from build123d import *

# Parameters (mm, degrees)
BOSS_EXTRUDE4_DEPTH                                 = 50
CBORE_FOR_00_BINDING_HEAD_MACHINE_SCREW_D           = 10.000000066
CBORE_FOR_00_BINDING_HEAD_MACHINE_SCREW_CBORE_D     = 19.999999878
CBORE_FOR_00_BINDING_HEAD_MACHINE_SCREW_CBORE_DEPTH = 3.000000096
BOSS_EXTRUDE5_REACH                                 = 119.883
SKETCH13_W                                          = 50
SKETCH13_H                                          = 2.915477917
BOSS_EXTRUDE5_DIRECTION_2_REACH                     = 119.883
CUT_EXTRUDE4_REACH                                  = 119.883
CUT_EXTRUDE4_DIRECTION_2_REACH                      = 119.883


with BuildPart() as part:
    # Sketch1 → Boss-Extrude4 (new body)
    with BuildSketch(Plane.XY):
        Polygon((-37.115898542, 15.206245128), (-57.115898542, 15.206245128), (-17.115898542, 75.206245128), (2.884101458, 75.206245128), (-13.756904429, 50.244736298), (-25.109531796, 50.244736298), (-40.64113729, 26.947328056), (-29.288509924, 26.947328056), align=None)
        Polygon((-77.115898542, 15.206245128), (-77.115898542, 75.206245128), (-17.115898542, 75.206245128), (-57.115898542, 15.206245128), align=None)
    extrude(amount=-BOSS_EXTRUDE4_DEPTH)

    # CBORE for #00 Binding Head Machine Screw2 (through all)
    with Locations(Plane.XY):
        with Locations((-57.115898542, 45.206245128)):
            CounterBoreHole(CBORE_FOR_00_BINDING_HEAD_MACHINE_SCREW_D / 2, CBORE_FOR_00_BINDING_HEAD_MACHINE_SCREW_CBORE_D / 2, CBORE_FOR_00_BINDING_HEAD_MACHINE_SCREW_CBORE_DEPTH)

    # Boss-Extrude5: up to this plane
    boss_extrude5_end = Plane(origin=(0, 50.244736298, -50), z_dir=(0, 1, 0))
    # Sketch13 → Boss-Extrude5 (add, up to the surface)
    with BuildSketch(Plane(origin=(3.425379126, 5.13806869, 0), x_dir=(0, 0, 1), z_dir=(0.5547001962252258, 0.8320502943378458, 0)), mode=Mode.PRIVATE) as boss_extrude5_sk1:
        with Locations((-25, -47.17806466)):
            Rectangle(SKETCH13_W, SKETCH13_H)
    boss_extrude5_tool1 = split(extrude(boss_extrude5_sk1.sketch, amount=BOSS_EXTRUDE5_REACH, mode=Mode.PRIVATE), bisect_by=boss_extrude5_end, keep=Keep.BOTH, mode=Mode.PRIVATE)
    add(boss_extrude5_tool1.solids().sort_by_distance((-35.829143, 31.30775, -25))[0])

    # Boss-Extrude5 direction 2: up to this plane
    boss_extrude5_direction_2_end = Plane(origin=(0, 26.947328056, -50), z_dir=(0, -1, 0))
    # Sketch13 → Boss-Extrude5 direction 2 (add, up to the surface)
    with BuildSketch(Plane(origin=(3.425379126, 5.13806869, 0), x_dir=(0, 0, 1), z_dir=(0.5547001962252258, 0.8320502943378458, 0)), mode=Mode.PRIVATE) as boss_extrude5_direction_2_sk1:
        with Locations((-25, -47.17806466)):
            Rectangle(SKETCH13_W, SKETCH13_H)
    boss_extrude5_direction_2_tool1 = split(extrude(boss_extrude5_direction_2_sk1.sketch, amount=-BOSS_EXTRUDE5_DIRECTION_2_REACH, mode=Mode.PRIVATE), bisect_by=boss_extrude5_direction_2_end, keep=Keep.BOTH, mode=Mode.PRIVATE)
    add(boss_extrude5_direction_2_tool1.solids().sort_by_distance((-35.829143, 31.30775, -25))[0])

    # Sketch13<5> → Cut-Extrude4 (cut, up to next)
    with BuildSketch(Plane(origin=(3.425379126, 5.13806869, 0), x_dir=(0, 0, 1), z_dir=(0.5547001962252258, 0.8320502943378458, 0)), mode=Mode.PRIVATE) as cut_extrude4_sk1:
        Polygon((-50, -39.317201463), (-30, -39.317201463), (-50, -45.720325701), align=None)
    cut_extrude4_tool1 = extrude(cut_extrude4_sk1.sketch, amount=-CUT_EXTRUDE4_REACH, mode=Mode.PRIVATE) & part.part
    # Sketch13<5> → Cut-Extrude4 (cut, up to next)
    with BuildSketch(Plane(origin=(3.425379126, 5.13806869, 0), x_dir=(0, 0, 1), z_dir=(0.5547001962252258, 0.8320502943378458, 0)), mode=Mode.PRIVATE) as cut_extrude4_sk2:
        Polygon((0, -39.317201463), (0, -45.720325701), (-20, -39.317201463), align=None)
    cut_extrude4_tool2 = extrude(cut_extrude4_sk2.sketch, amount=-CUT_EXTRUDE4_REACH, mode=Mode.PRIVATE) & part.part
    add(cut_extrude4_tool1.solids().sort_by_distance((-31.064417, 28.131266, -43.333333))[0], mode=Mode.SUBTRACT)
    add(cut_extrude4_tool2.solids().sort_by_distance((-31.064417, 28.131266, -6.666667))[0], mode=Mode.SUBTRACT)

    # Sketch13<5> → Cut-Extrude4 direction 2 (cut, up to next)
    with BuildSketch(Plane(origin=(3.425379126, 5.13806869, 0), x_dir=(0, 0, 1), z_dir=(0.5547001962252258, 0.8320502943378458, 0)), mode=Mode.PRIVATE) as cut_extrude4_direction_2_sk1:
        Polygon((-50, -39.317201463), (-30, -39.317201463), (-50, -45.720325701), align=None)
    cut_extrude4_direction_2_tool1 = extrude(cut_extrude4_direction_2_sk1.sketch, amount=CUT_EXTRUDE4_DIRECTION_2_REACH, mode=Mode.PRIVATE) & part.part
    # Sketch13<5> → Cut-Extrude4 direction 2 (cut, up to next)
    with BuildSketch(Plane(origin=(3.425379126, 5.13806869, 0), x_dir=(0, 0, 1), z_dir=(0.5547001962252258, 0.8320502943378458, 0)), mode=Mode.PRIVATE) as cut_extrude4_direction_2_sk2:
        Polygon((0, -39.317201463), (0, -45.720325701), (-20, -39.317201463), align=None)
    cut_extrude4_direction_2_tool2 = extrude(cut_extrude4_direction_2_sk2.sketch, amount=CUT_EXTRUDE4_DIRECTION_2_REACH, mode=Mode.PRIVATE) & part.part
    add(cut_extrude4_direction_2_tool1.solids().sort_by_distance((-31.064417, 28.131266, -43.333333))[0], mode=Mode.SUBTRACT)
    add(cut_extrude4_direction_2_tool2.solids().sort_by_distance((-31.064417, 28.131266, -6.666667))[0], mode=Mode.SUBTRACT)


solid = part.part
For this review, take the finished solid that the model builds, in its own axes (mm). A direction names the side the tool comes from. Give positions to 0.01 mm unless a question says otherwise; leave off trailing zeros. Order: outer loops, then holes, each group sorted by start corner. A loop starts at its lowest first (then second) coordinate and runs counter-clockwise, first axis right, second up. Notation, with made-up numbers: M 25,4 L 37,4 A17 ccw 37,22 Z; hole C 69.5,25 d7. An arc over 180 degrees is marked long. Answer in a Markdown table with one row per item. Add a question column.
(1) For faces 4 (the face through (-37.016, 21.209, -9.86)), 5 (the face through (-18, 50.245, -25)), 6 (the face through (-55, 50, -3)), list the 3-axis set-ups (+Z, -Z, +X, -X, +Y, -Y) from which the entire face can be reached by the end or side of a thin tool; tool diameter is ignored.
(2) For pin 1 (3 mm diameter, centred on x = -48.5, y = 62, fed in from +Z); pin 2 (4 mm diameter, centred on x = -16, z = -34, fed in from -Y); pin 3 (5 mm diameter, centred on y = 60.5, z = -22.5, fed in from +X), all flat-tipped, find the tip position at first contact; note any pin that passes through.
(3) Wall thickness on probe 1 along X at (y, z) = (48.5, -10); probe 2 along Y at (x, z) = (-57.5, -17); probe 3 along X at (y, z) = (37.5, -4): over which ranges is each line inside the solid? List them lowest first. Write a range as [from, to].
(4) Consider section D-D on y = 53.5. State the section outline as (x, z) points.
(5) Consider section C-C on z = -13. State the section outline as (x, y) points.
(6) Mouldability with a two-part tool opening along Y and no side actions: class faces 1 (the face through (-33.147, 21.159, -24.93)), 2 (the face through (-29.11, 38.76, -25.35)), 3 (the face through (-49, 51, -50)) as +Y half, -Y half, draft (parallel to the pull), parting line (faces both ways), or undercut.
(7) Consider section A-A on x = -57.5. State the section outline as (y, z) points, and give its area (3 significant figures).
(8) Consider section B-B on y = 44. State the section outline as (x, z) points, and give its area (3 significant figures).
Evaluation:
| question | item | result |
|---|---|---|
| 1 | face 4 | +Z, +X, -Y |
| 1 | face 5 | +Z, -Z, +X, -Y |
| 1 | face 6 | +Z |
| 2 | pin 1 | stops at z = 0 |
| 2 | pin 2 | stops at y = 50.24 |
| 2 | pin 3 | stops at x = -5.25 |
| 3 | probe 1 | x = [-77.12, -60.88], [-53.35, -26.27], [-26.12, -22.62] |
| 3 | probe 2 | y = [15.21, 40.22], [50.19, 75.21] |
| 3 | probe 3 | x = [-77.12, -33.61], [-33.45, -29.95] |
| 4 | outline | M -77.12,-50 L -19.28,-50 L -11.59,-30 L -11.59,-20 L -19.28,0 L -51.53,0 L -51.53,-3 L -62.7,-3 L -62.7,0 L -77.12,0 Z |
| 5 | outline | M -77.12,15.21 L -39.81,15.21 L -31.98,26.95 L -36.98,26.95 L -21.45,50.24 L -16.45,50.24 L 0.19,75.21 L -77.12,75.21 Z; hole C -57.12,45.21 d10; hole M -40.64,26.95 L -40.49,26.95 L -24.96,50.24 L -25.11,50.24 Z |
| 6 | face 1 | -Y half |
| 6 | face 2 | undercut |
| 6 | face 3 | draft |
| 7 | outline | M 15.21,-50 L 40.22,-50 L 40.22,-3 L 35.21,-3 L 35.21,0 L 15.21,0 Z; M 50.19,-50 L 75.21,-50 L 75.21,0 L 55.2,0 L 55.2,-3 L 50.19,-3 Z |
| 7 | area | 2,470 mm^2 |
| 8 | outline | M -77.12,-50 L -61.97,-50 L -61.97,-3 L -67.04,-3 L -67.04,0 L -77.12,0 Z; M -52.26,-50 L -29.27,-50 L -29.27,0 L -47.19,0 L -47.19,-3 L -52.26,-3 Z; M -29.12,-50 L -25.62,-50 L -25.62,0 L -29.12,0 Z |
| 8 | area | 2,050 mm^2 |
